For this review, take the finished solid that the model builds, in its own axes (mm). A direction names the side the tool comes from. Coordinates: 2 decimals unless noted, no trailing zeros. Loops run counter-clockwise (first coordinate to the right, second up) from the corner with the lowest first, then second, coordinate; pieces in that order, holes last. Notation, with made-up numbers: (80, -30) -> (139, -30) arc R30 cw to (139, -8) -> close; hole circle Ø4 at (-12, 39.25). An arc over 180 degrees is marked (long way). One line per item, written item: value.
from build123d import *

# Parameters (mm, degrees)
SKETCH_1_W          = 20
SKETCH_1_H          = 18
EXTRUDE_1_DEPTH     = 5
SKETCH_2_R          = 6.5
CUT_EXTRUDE_1_DEPTH = 28.367864367
SKETCH_3_W          = 2.6
SKETCH_3_H          = 18
EXTRUDE_2_DEPTH     = 2
SKETCH_4_R          = 1
CUT_EXTRUDE_2_DEPTH = 28.802877549
CUT_EXTRUDE_3_DEPTH = 28.802877621
SKETCH_6_W          = 5
SKETCH_6_H          = 3
EXTRUDE_3_DEPTH     = 4
SKETCH_7_R          = 1
CUT_EXTRUDE_4_DEPTH = 28.802877621


with BuildPart() as part:
    # 草图1 → 凸台-拉伸1 (new body)
    with BuildSketch(Plane(origin=(0, 0, 0), x_dir=(0, 0, -1), z_dir=(1, 0, 0))):
        with Locations((10, -9)):
            Rectangle(SKETCH_1_W, SKETCH_1_H)
    extrude(amount=EXTRUDE_1_DEPTH)

    # 草图2 → 切除-拉伸1 (cut, through all)
    with BuildSketch(Plane(origin=(5, 0, 0), x_dir=(0, 0, -1), z_dir=(1, 0, 0))):
        with Locations((10, -9)):
            Circle(SKETCH_2_R)
    extrude(amount=-CUT_EXTRUDE_1_DEPTH, mode=Mode.SUBTRACT)

    # 草图3 → 凸台-拉伸2 (add)
    with BuildSketch(Plane(origin=(5, 0, 0), x_dir=(0, 0, -1), z_dir=(1, 0, 0))):
        with Locations((1.3, -9)):
            Rectangle(SKETCH_3_W, SKETCH_3_H)
        with Locations((18.7, -9)):
            Rectangle(SKETCH_3_W, SKETCH_3_H)
    extrude(amount=EXTRUDE_2_DEPTH)

    # 草图4 → 切除-拉伸2 (cut, through all)
    with BuildSketch(Plane.XY):
        with Locations((4.5, -9)):
            Circle(SKETCH_4_R)
    extrude(amount=-CUT_EXTRUDE_2_DEPTH, mode=Mode.SUBTRACT)

    # 草图5 → 切除-拉伸3 (cut, through all)
    with BuildSketch(Plane.XY):
        Polygon((7, 0), (2, 0), (7, -6.5), align=None)
        Polygon((7, -18), (7, -11.5), (2, -18), align=None)
    extrude(amount=-CUT_EXTRUDE_3_DEPTH, mode=Mode.SUBTRACT)

    # 草图6 → 凸台-拉伸3 (add)
    with BuildSketch(Plane.ZY):
        with Locations((-17.5, -16.5)):
            Rectangle(SKETCH_6_W, SKETCH_6_H)
        with Locations((-17.5, -1.5)):
            Rectangle(SKETCH_6_W, SKETCH_6_H)
        with Locations((-2.5, -1.5)):
            Rectangle(SKETCH_6_W, SKETCH_6_H)
        with Locations((-2.5, -16.5)):
            Rectangle(SKETCH_6_W, SKETCH_6_H)
    extrude(amount=EXTRUDE_3_DEPTH)

    # 草图7 → 切除-拉伸4 (cut, through all)
    with BuildSketch(Plane(origin=(0, 0, 0), x_dir=(1, 0, 0), z_dir=(0, 1, 0))):
        with Locations(Location((-1, 17.5, 0), (0, 0, 270))):
            Circle(SKETCH_7_R)
        with Locations(Location((-1, 2.5, 0), (0, 0, 270))):
            Circle(SKETCH_7_R)
    extrude(amount=-CUT_EXTRUDE_4_DEPTH, mode=Mode.SUBTRACT)


solid = part.part
1. To check wall thickness, follow probe 1 along Z at (x, y) = (-1, -0.75); probe 2 along Z at (x, y) = (-1.75, -16.75); probe 3 along X at (y, z) = (-9, -18). State the ranges of each line that lie inside material, in increasing order. Write a range as from..to.
Return value:
probe 1: z = -20..-18.5, -16.5..-15, -5..-3.5, -1.5..0
probe 2: z = -20..-18.16, -16.84..-15, -5..-3.16, -1.84..0
probe 3: x = 0..3.5, 5.5..7
2. Take a section at D-D, the plane z = -18. Give the boundary of the cut face in (x, y).
Return value:
outline: (-4, -18) -> (-1.87, -18) -> (-1.87, -15) -> (-4, -15) -> close; (-4, -3) -> (-1.87, -3) -> (-1.87, 0) -> (-4, 0) -> close; (-0.13, -18) -> (2, -18) -> (7, -11.5) -> (7, -6.5) -> (2, 0) -> (-0.13, 0) -> (-0.13, -3) -> (0, -3) -> (0, -15) -> (-0.13, -15) -> close; hole circle Ø2 at (4.5, -9)
3. Take a section at A-A, the plane x = -1. Give the number of separate pieces and of enclosed holes in the cut face, and give its area (3 significant figures).
Return value:
separate pieces: 8
enclosed holes: 0
area: 36.0 mm2
4. Insertion check: pin 1 Ø1 at (y, z) = (-12, -4) entering from +X. The pin has a flat end and moves straight along its axis. Give the tip position at first contact, or say it passes through.
Return value:
pin 1: stops at x = 5
5. Take a section at B-B, the plane z = -9.75. Give the boundary of the cut face in (x, y).
Return value:
outline: (0, -18) -> (2, -18) -> (3.93, -15.5) -> (0, -15.5) -> close; (0, -2.5) -> (3.93, -2.5) -> (2, 0) -> (0, 0) -> close
6. Take a section at C-C, the plane y = -10.25. Give the boundary of the cut face in (x, z), and give its area (3 significant figures).
Return value:
outline: (0, -20) -> (7, -20) -> (7, -17.4) -> (5, -17.4) -> (5, -16.38) -> (0, -16.38) -> close; (0, -3.62) -> (5, -3.62) -> (5, -2.6) -> (7, -2.6) -> (7, 0) -> (0, 0) -> close
area: 46.6 mm2
7. For faces 4 (the flat face through (-2.4, -15, -2.5)), 5 (the flat face through (0.4, -18, -10.1)), 6 (the cylindrical face through (2.54, -7.05, -16.2)), 7 (the flat face through (6, -9, -17.4)), 8 (the flat face through (-2, -2, -5)), list the 3-axis set-ups (+Z, -Z, +X, -X, +Y, -Y) from which the entire face can be reached by the end or side of a thin tool; tool diameter is ignored.
Return value:
face 4: +Z, -Z, -X
face 5: +Z, -Z, +X, -X, -Y
face 6: +X, -X
face 7: +X, +Y, -Y
face 8: -X, +Y, -Y
8. The part is to be moulded in two halves that separate along Z. For faces 1 (the flat face through (1, -9, 0)), 2 (the flat face through (3.354, -1.76, -9.86)), 3 (the flat face through (5, -6, -4)), say which applies: pulls with the +Z half, pulls with the -Z half, needs draft (parallel to the pull), parting line crosses it, or undercut.
Return value:
face 1: pulls with the +Z half
face 2: needs draft
face 3: undercut
